```python
from build123d import *

# Parameters (mm, degrees)
F0_W     = 176.5
F0_H     = 116
F1_DEPTH = 6
F2_SIZE  = 10
F4_R     = 2
F3_R     = 50.125
F3_R_2   = 44.875
F5_DEPTH = 3
F3_R_3   = 1.25
F6_DEPTH = 6.001
F7_R     = 5
F8_DEPTH = 4


with BuildPart() as f1:
    # F0 (on Top) → F1 (new body)
    with BuildSketch(Plane.XY):
        with Locations((-3.4001671076, 29.7604629695)):
            Rectangle(F0_W, F0_H)
    extrude(amount=F1_DEPTH)

    # F2
    f2_edges = [f1.edges().sort_by_distance(p)[0] for p in [
        (-91.650167, -28.239537, 3),
        (84.849833, -28.239537, 3),
        (84.849833, 87.760463, 3),
        (-91.650167, 87.760463, 3),
    ]]
    chamfer(f2_edges, length=F2_SIZE)

    # F4
    f4_edges = [f1.edges().sort_by_distance(p)[0] for p in [
        (-3.400167, -28.239537, 6),
        (-86.650167, -23.239537, 6),
        (-91.650167, 29.760463, 6),
        (-86.650167, 82.760463, 6),
        (-3.400167, 87.760463, 6),
        (79.849833, 82.760463, 6),
        (84.849833, 29.760463, 6),
        (79.849833, -23.239537, 6),
        (-81.650167, -28.239537, 3),
        (-91.650167, -18.239537, 3),
        (-91.650167, 77.760463, 3),
        (-81.650167, 87.760463, 3),
        (74.849833, 87.760463, 3),
        (84.849833, 77.760463, 3),
        (84.849833, -18.239537, 3),
        (74.849833, -28.239537, 3),
    ]]
    fillet(f4_edges, radius=F4_R)

    # F3 (on face) → F5 (cut)
    with BuildSketch(Plane.XY.offset(6)):
        with Locations((-3.4001671076, 29.7604629695)):
            Circle(F3_R)
        with Locations((-3.4001671076, 29.7604629695)):
            Circle(F3_R_2, mode=Mode.SUBTRACT)
    extrude(amount=-F5_DEPTH, mode=Mode.SUBTRACT)

    # F3 (on face) → F6 (cut, through all)
    with BuildSketch(Plane.XY.offset(6)):
        with Locations((-3.4001671076, 29.7604629695)):
            Circle(F3_R_3)
    extrude(amount=-F6_DEPTH, mode=Mode.SUBTRACT)

    # F7 (on face) → F8 (cut)
    with BuildSketch(Plane(origin=(0, 0, 0), x_dir=(1, 0, 0), z_dir=(0, 0, -1))):
        with Locations((-3.4001671076, -29.7604629695)):
            Circle(F7_R)
    extrude(amount=-F8_DEPTH, mode=Mode.SUBTRACT)


solid = f1.part
```
Can you work these out from the model? Positions are in its coordinate system, mm. A direction names the side the tool comes from. Coordinates: 2 decimals unless noted, no trailing zeros. Loops run counter-clockwise (first coordinate to the right, second up) from the corner with the lowest first, then second, coordinate; pieces in that order, holes last.
Item 1: Suppose I cut it at B-B (y = 43.5). Please give me the cut outline in (x, z), then the cut area to 3 significant figures.
Answers below:
outline: (-91.65, 0) - (84.85, 0) - (84.85, 4) arc R2 ccw to (82.85, 6) - (44.81, 6) - (44.81, 3) - (39.32, 3) - (39.32, 6) - (-46.12, 6) - (-46.12, 3) - (-51.61, 3) - (-51.61, 6) - (-89.65, 6) arc R2 ccw to (-91.65, 4) - close
area: 1,020 mm2
Item 2: If we mould it in two halves opening along Y, with no side actions, what happens to faces 4 (the face through (-4, 20, 6)), 5 (the face through (-4, 87.76, 2)), 6 (the face through (-2, 31, 4))? For each: released by +Y, released by -Y, zero draft, split by the parting line, or undercut.
Answers below:
face 4: zero draft
face 5: released by +Y
face 6: undercut
Item 3: Suppose I cut it at D-D (y = 26.5). Please give me the cut outline in (x, z).
Answers below:
outline: (-91.65, 0) - (-7.19, 0) - (-7.19, 4) - (0.39, 4) - (0.39, 0) - (84.85, 0) - (84.85, 4) arc R2 ccw to (82.85, 6) - (46.62, 6) - (46.62, 3) - (41.36, 3) - (41.36, 6) - (-48.16, 6) - (-48.16, 3) - (-53.42, 3) - (-53.42, 6) - (-89.65, 6) arc R2 ccw to (-91.65, 4) - close
Item 4: Please list where these lines run through material, in increasing order: L1, parallel to Y at x = 7, z = 4.45; L2, parallel to X at y = 34, z = 5; L3, parallel to X at y = 41, z = 5.65.
Answers below:
L1: y = -28.19 to -19.27, -13.89 to 73.41, 78.79 to 87.71
L2: x = -91.38 to -53.35, -48.07 to 41.27, 46.55 to 84.58
L3: x = -90.78 to -52.25, -46.84 to 40.04, 45.45 to 83.98
Item 5: Suppose I cut it at A-A (z = 5.1). State how many separate pieces and enclosed holes the cut face has, then the cut area to 3 significant figures.
Answers below:
separate pieces: 2
enclosed holes: 2
area: 18,500 mm2
Item 6: Suppose I cut it at C-C (x = -37). Please give me the cut outline in (y, z).
Answers below:
outline: (-28.24, 0) - (87.76, 0) - (87.76, 4) arc R2 ccw to (85.76, 6) - (66.96, 6) - (66.96, 3) - (59.51, 3) - (59.51, 6) - (0.01, 6) - (0.01, 3) - (-7.44, 3) - (-7.44, 6) - (-26.24, 6) arc R2 ccw to (-28.24, 4) - close
Item 7: I'm going to push a flat-ended pin straight in: pin 1 (3 mm diameter, centred on x = -2, y = 30, fed in from -Z). Where does the tip first touch, or does it pass through?
Answers below:
pin 1: stops at z = 4
Item 8: Which directions (+Z, -Z, +X, -X, +Y, -Y) give clear straight access to the entire face, cutting with the end or side of a thin tool? Please do faces 1 (the face through (-13.128, -14.047, 4.521)), 2 (the face through (-86.59, 82.82, 1.97)), 3 (the face through (-4.051, 24.803, 1.972)).
Answers below:
face 1: +Z
face 2: +Z, -Z, -X, +Y
face 3: -Z
